Design review of the part built by this model. Coordinates are the model's own, in mm. A direction names the side the tool comes from. Coordinates: 2 decimals unless noted, no trailing zeros. Loops run counter-clockwise (first coordinate to the right, second up) from the corner with the lowest first, then second, coordinate; pieces in that order, holes last. Notation, with made-up numbers: M -24.75,-2 L -15.75,-2 A30 cw -15.75,36 Z; hole C -16.75,-39.75 d11. An arc over 180 degrees is marked long. Answer as a JSON object with one key per item and string values. Group by question number.
1. Consider section C-C (z = -6.25). State the section outline as (x, y) points, then the cut area to 3 significant figures.
2. Consider section D-D (y = -8). Count the separate pieces of the cut face and the enclosed holes in it, then the cut area to 3 significant figures.
3. To check wall thickness, follow probe 1 along Y at (x, z) = (0, -4.75); probe 2 along Y at (x, z) = (0, -1.5); probe 3 along X at (y, z) = (-8, -3.75). State the ranges of each line that lie inside material, in increasing order.
4. Insertion check: pin 1 (4 mm diameter, centred on x = 13.86, y = 8, fed in from +Z); pin 2 (2 mm diameter, centred on y = 11.5, z = -6, fed in from -X); pin 3 (1 mm diameter, centred on x = 4.5, z = -5.5, fed in from -Y); pin 4 (1 mm diameter, centred on x = 7, z = -4, fed in from +Y). Each pin has a flat end and moves straight along its axis. Give the tip position at first contact, or say it passes through.
5. Consider section B-B (y = 0). State the section outline as (x, z) points.
6. Machinability: for faces 1 (the cylindrical face through (19.524, -4.336, -2.479)), 2 (the flat face through (9, 9, -7)), which of the approach directions +Z, -Z, +X, -X, +Y, -Y give a long, thin tool a straight path to every point of the face, cutting with its end or side? Answer none if there is none.
7. Draft analysis for pull direction Y (two halves, no side actions). For faces 3 (the flat face through (18, 10, -4)), 4 (the cylindrical face through (12.8, -6.8, -3.5)), 5 (the cylindrical face through (21.477, -4.769, -5.479)), state which applies: +Y half, -Y half, draft (parallel to the pull), parting line (faces both ways), or undercut.
8. Consider section A-A (x = 0). State the section outline as (y, z) points.
Autodesk Inventor part; units mm, degrees
ref_plane "YZ Plane" through (0, 0, 0) normal (1, 0, 0) x (0, 1, 0)
ref_plane "XZ Plane" through (0, 0, 0) normal (0, 1, 0) x (-1, 0, 0)
ref_plane "XY Plane" through (0, 0, 0) normal (0, 0, 1) x (1, 0, 0)
sketch "スケッチ1" plane through (0, 0, 0) normal (1, 0, 0) x (0, 1, 0)
  line L0 (12, 0) -> (12, -7)
  line L1 (22, -7) -> (22, -4)
  line L2 (22, -4) -> (20, -4)
  line L3 (20, -4) -> (20, 0)
  line L4 (20, 0) -> (12, 0)
  line L5 (0, -8.4) -> (0, 1.4)
  line L6 (22, -7) -> (12, -7)
  point P0 (0, 0)
  dimension "d0" = 20
  dimension "d1" = 2
  dimension "d2" = 4
  dimension "d3" = 3
  dimension "d4" = 8
revolve "回転1" add sketch "スケッチ1" angle 360 about axis through (0, 0, -10) along (0, 0, 1)
sketch "スケッチ2" plane through (0, 0, 0) normal (0, 0, 1) x (1, 0, 0)
  circle A0 centre (0, 0) radius 20
  circle A1 centre (0, 0) radius 16
  point P0 (0, 16)
  point P1 (-13.8564, 8)
  point P2 (-13.8564, -8)
  point P3 (0, -16)
  point P4 (13.8564, -8)
  point P5 (13.8564, 8)
  dimension "d8" = 4
  dimension "d11" = 360
hole "穴1" at (0, 16, 0) at (-13.8564, 8, 0) at (-13.8564, -8, 0) at (0, -16, 0) at (13.8564, -8, 0) at (13.8564, 8, 0) direction (0, 0, -1) diameter 3.2 end through all
chamfer "面取り1" distance 1 angle 45 1 edges at (0, -20, 0)
properties part number "base11" material "ABS プラスチック"
Findings below:
{
 "1": {"outline": "C 0,0 d44; hole C -13.86,-8 d3.2; hole C -13.86,8 d3.2; hole C 0,0 d24; hole C 0,-16 d3.2; hole C 0,16 d3.2; hole C 13.86,-8 d3.2; hole C 13.86,8 d3.2", "area": "1,020 mm^2"},
 "2": {"separate pieces": "4", "enclosed holes": "0", "area": "98.5 mm^2"},
 "3": {"probe 1": "y = -22 to -17.6, -14.4 to -12, 12 to 14.4, 17.6 to 22", "probe 2": "y = -20 to -17.6, -14.4 to -12, 12 to 14.4, 17.6 to 20", "probe 3": "x = -18.33 to -15.46, -12.26 to -8.94, 8.94 to 12.26, 15.46 to 18.33"},
 "4": {"pin 1": "stops at z = 0", "pin 2": "stops at x = -19.33", "pin 3": "stops at y = -21.63", "pin 4": "stops at y = 21.02"},
 "5": {"outline": "M -22,-7 L -12,-7 L -12,0 L -19,0 L -20,-1 L -20,-4 L -22,-4 Z; M 12,-7 L 22,-7 L 22,-4 L 20,-4 L 20,-1 L 19,0 L 12,0 Z"},
 "6": {"face 1": "+Z", "face 2": "-Z, +X, -X, +Y, -Y"},
 "7": {"face 3": "draft", "face 4": "undercut", "face 5": "parting line"},
 "8": {"outline": "M -22,-7 L -17.6,-7 L -17.6,0 L -19,0 L -20,-1 L -20,-4 L -22,-4 Z; M -14.4,-7 L -12,-7 L -12,0 L -14.4,0 Z; M 12,-7 L 14.4,-7 L 14.4,0 L 12,0 Z; M 17.6,-7 L 22,-7 L 22,-4 L 20,-4 L 20,-1 L 19,0 L 17.6,0 Z"}
}
